```python
from build123d import *

# Parameters (mm, degrees)
SKETCH_1_R      = 10
EXTRUDE_1_DEPTH = 3
SKETCH_2_R      = 3
EXTRUDE_2_DEPTH = 20


with BuildPart() as part:
    # 草图1 → 凸台-拉伸1 (new body)
    with BuildSketch(Plane(origin=(0, 0, 0), x_dir=(1, 0, 0), z_dir=(0, 1, 0))):
        with Locations(Location((0, 0, 0), (0, 0, 270))):
            Circle(SKETCH_1_R)
    extrude(amount=EXTRUDE_1_DEPTH)

    # 草图2 → 凸台-拉伸2 (add)
    with BuildSketch(Plane(origin=(0, 3, 0), x_dir=(1, 0, 0), z_dir=(0, 1, 0))):
        with Locations(Location((0, 0, 0), (0, 0, 270))):
            Circle(SKETCH_2_R)
    extrude(amount=EXTRUDE_2_DEPTH)

    # 草图3 → 旋转2 (revolve)
    with BuildSketch(Plane.XY, mode=Mode.PRIVATE) as revolve_2_sk:
        with BuildLine():
            Line((-10, 3), (-3, 3))
            Line((-3, 3), (-3, 13))
            ThreePointArc((-3, 13), (-4.923888846, 6.896722192), (-10, 3))
        make_face()
    revolve(revolve_2_sk.sketch.rotate(Axis((0, -1000, 0), (0, 1, 0)), 180), axis=Axis((0, -1000, 0), (0, 1, 0)))


solid = part.part
```
Read the model definition and answer for the solid it produces. Units are mm, in the model's axes. A direction names the side the tool comes from. Coordinates: 2 decimals unless noted, no trailing zeros. Write each loop counter-clockwise with the first axis right and the second up, starting at its lowest first coordinate (ties: lowest second). Pieces come first, ordered by that corner, then holes. Notation, with made-up numbers: (36.25, -24) -> (55.25, -24) arc R32 cw to (55.25, 6) -> close; hole circle Ø6 at (34, -10.75). An arc over 180 degrees is marked (long way). Answer as a JSON object with one key per item and string values.
Q1. The part is cut by section C-C on y = 20. Give the vertices of the cut face in (x, z), then the cut area to 3 significant figures.
The answers:
{"outline": "circle Ø6 at (0, 0)", "area": "28.3 mm2"}
Q2. Consider line 1 (X direction, y = 19.25, z = 1.25); line 2 (X direction, y = 6.5, z = -1.5); line 3 (Z direction, x = -4.75, y = 2.5). Determine where each line is inside the solid, lowest interval first. Write a range as [from, to].
The answers:
{"line 1": "x = [-2.73, 2.73]", "line 2": "x = [-5, 5]", "line 3": "z = [-8.8, 8.8]"}
Q3. A tool of negligible diameter and unlimited length cuts with its end or side. For faces 1 (the cylindrical face through (0.9, 17.93, 2.86)), 2 (the cylindrical face through (-9.76, 1.48, -2.17)), from which of +Z, -Z, +X, -X, +Y, -Y can it reach the whole face along a straight path? Write none if from no direction.
The answers:
{"face 1": "+Y", "face 2": "+Y, -Y"}
Q4. The part is cut by section D-D on y = 8. Give the vertices of the cut face in (x, z).
The answers:
{"outline": "circle Ø8.5 at (0, 0)"}
Q5. Flat-ended cylindrical pins translate along their axes: pin 1 Ø4 at (y, z) = (8.5, -2) entering from -X; pin 2 Ø12 at (x, y) = (5, 8.5) entering from +Z; pin 3 Ø5 at (x, y) = (2.5, 8.5) entering from -Z. Find the tip coordinate at first contact, or state that the pin passes through.
The answers:
{"pin 1": "stops at x = -4.95", "pin 2": "stops at z = 9.66", "pin 3": "stops at z = -5.24"}
Q6. The part is cut by section B-B on x = 0. Give the vertices of the cut face in (y, z).
The answers:
{"outline": "(0, -10) -> (3, -10) arc R10.64 cw to (13, -3) -> (23, -3) -> (23, 3) -> (13, 3) arc R10.64 cw to (3, 10) -> (0, 10) -> close"}
Q7. The part is cut by section A-A on z = 0. Give the vertices of the cut face in (x, y), then the cut area to 3 significant figures.
The answers:
{"outline": "(-10, 0) -> (10, 0) -> (10, 3) arc R10.64 cw to (3, 13) -> (3, 23) -> (-3, 23) -> (-3, 13) arc R10.64 cw to (-10, 3) -> close", "area": "218 mm2"}
